```python
from build123d import *

# Parameters (mm, degrees)
SKETCH1_R                = 12.5
CORPO_DEPTH              = 3
SKETCH2_R                = 11.5
SKETCH2_R_2              = 8.5
EIXO_DE_ENCAIXE_20_DEPTH = 2.5
CHANFRO_1X45_SIZE        = 1


with BuildPart() as part:
    # Sketch1 → Corpo (new body)
    with BuildSketch(Plane.XY):
        Circle(SKETCH1_R)
    extrude(amount=-CORPO_DEPTH)

    # Sketch2 → Eixo de Encaixe - Ø20 (add)
    with BuildSketch(Plane(origin=(0, 0, -3), x_dir=(-1, 0, 0), z_dir=(0, 0, -1))):
        with Locations(Location((0, 0, 0), (0, 0, 180))):
            Circle(SKETCH2_R)
        Circle(SKETCH2_R_2, mode=Mode.SUBTRACT)
    extrude(amount=EIXO_DE_ENCAIXE_20_DEPTH)

    # Chanfro 1x45°
    chanfro_1x45_edges = [part.edges().sort_by_distance(p)[0] for p in [
        (-12.5, 0, 0),
        (-11.5, 0, -5.5),
        (8.5, 0, -5.5),
    ]]
    chamfer(chanfro_1x45_edges, length=CHANFRO_1X45_SIZE)


solid = part.part
```
Input: part model. Units: mm. Frame: model coordinates. A direction names the side the tool comes from. Round coordinates to 2 decimals unless told otherwise and drop trailing zeros. Loops run counter-clockwise (first coordinate to the right, second up) from the corner with the lowest first, then second, coordinate; pieces in that order, holes last. Notation, with made-up numbers: (-1, -31.75) -> (10, -31.75) arc R21 ccw to (10, -14.75) -> close; hole circle Ø6 at (-37, 24). An arc over 180 degrees is marked (long way). Write each question's results on one line, items separated by ' | '.
1. First-contact query: P1, Ø2, axis at x = -6.5, z = -3, coming from the +Y side (3 decimals); P2, Ø1.5, axis at x = 3.5, z = -4, coming from the -Y side. Flat tips, straight axial feed; report the tip coordinate or a pass-through.
Geometry results:
P1: y = 11.225 | P2: y = -11.17
2. Set-up query: faces 4 (the face through (-5, 9, -5.5)), 5 (the face through (0, 0, -3)). Return all of +Z, -Z, +X, -X, +Y, -Y with unobstructed straight access to the full face (end or side cutting, diameter ignored); none if empty.
Geometry results:
face 4: -Z, +X, -X, +Y, -Y | face 5: -Z
3. Section A-A (x = 0). Return loops of the section in (y, z).
Geometry results:
outline: (-12.5, -3) -> (-11.5, -3) -> (-11.5, -4.5) -> (-10.5, -5.5) -> (-9.5, -5.5) -> (-8.5, -4.5) -> (-8.5, -3) -> (8.5, -3) -> (8.5, -4.5) -> (9.5, -5.5) -> (10.5, -5.5) -> (11.5, -4.5) -> (11.5, -3) -> (12.5, -3) -> (12.5, -1) -> (11.5, 0) -> (-11.5, 0) -> (-12.5, -1) -> close
4. Section C-C (z = -2.1). Return loops of the section in (x, y), and give its area (3 significant figures).
Geometry results:
outline: circle Ø25 at (0, 0) | area: 491 mm2
5. Mould query, pull axis X, two halves, no side actions, for faces 1 (the face through (0, 0, 0)), 2 (the face through (-4.57, 7.167, -3.74)), 3 (the face through (11.923, 3.755, -1.986)). Classes: +X half, -X half, draft (parallel to the pull), parting line (faces both ways), or undercut.
Geometry results:
face 1: draft | face 2: undercut | face 3: parting line
6. Ray query, line 1 (Y direction, x = 0, z = -3.8); line 2 (Z direction, x = 2.25, y = -6.75); line 3 (Y direction, x = -6.25, z = -4.85). Return the intervals inside material, ascending. Write a range as from..to.
Geometry results:
line 1: -11.5..-8.5, 8.5..11.5 | line 2: -3..0 | line 3: -9.23..-6.27, 6.27..9.23
7. Section D-D (z = -3.5). Return loops of the section in (x, y), and give its area (3 significant figures).
Geometry results:
outline: circle Ø23 at (0, 0); hole circle Ø17 at (0, 0) | area: 188 mm2
